from build123d import *

# Parameters (mm, degrees)
SKETCH1_R             = 2.6
BOSS_EXTRUDE1_DEPTH   = 1.6
SKETCH2_R             = 3.45
BOSS_EXTRUDE2_DEPTH   = 1.4
M5X0_8_TAPPED_HOLE1_D = 4.2


with BuildPart() as part:
    # Sketch1 → Boss-Extrude1 (new body)
    with BuildSketch(Plane.XY):
        with BuildLine():
            Line((-2.5, 7.216878365), (2.5, 7.216878365))
            Line((2.5, 7.216878365), (26.315698604, 20.966878365))
            Line((26.315698604, 20.966878365), (29.903623675, 21.701093146))
            ThreePointArc((29.903623675, 21.701093146), (30.819646028, 21.599539147), (31.503382336, 20.981546567))
            Line((31.503382336, 20.981546567), (33.922243506, 16.791956125))
            ThreePointArc((33.922243506, 16.791956125), (34.115572625, 15.890826823), (33.745509792, 15.046751195))
            Line((33.745509792, 15.046751195), (31.315698604, 12.306624327))
            Line((31.315698604, 12.306624327), (7.5, -1.443375673))
            Line((7.5, -1.443375673), (9.220577137, -4.423502692))
            ThreePointArc((9.220577137, -4.423502692), (9.220577137, -5.323502692), (8.441154273, -5.773502692))
            Line((8.441154273, -5.773502692), (-8.441154273, -5.773502692))
            ThreePointArc((-8.441154273, -5.773502692), (-9.220577137, -5.323502692), (-9.220577137, -4.423502692))
            Line((-9.220577137, -4.423502692), (-7.5, -1.443375673))
            Line((-7.5, -1.443375673), (-31.315698604, 12.306624327))
            Line((-31.315698604, 12.306624327), (-33.745509792, 15.046751195))
            ThreePointArc((-33.745509792, 15.046751195), (-34.115572625, 15.890826823), (-33.922243506, 16.791956125))
            Line((-33.922243506, 16.791956125), (-31.503382336, 20.981546567))
            ThreePointArc((-31.503382336, 20.981546567), (-30.819646028, 21.599539147), (-29.903623675, 21.701093146))
            Line((-29.903623675, 21.701093146), (-26.315698604, 20.966878365))
            Line((-26.315698604, 20.966878365), (-2.5, 7.216878365))
        make_face()
        Circle(SKETCH1_R, mode=Mode.SUBTRACT)
    extrude(amount=BOSS_EXTRUDE1_DEPTH)

    # Sketch2 → Boss-Extrude2 (add)
    with BuildSketch(Plane.XY.offset(1.6)):
        with Locations((26.621620912, 15.37)):
            Circle(SKETCH2_R)
        with Locations((9.301112837, 5.37)):
            Circle(SKETCH2_R)
        with Locations((-9.301112837, 5.37)):
            Circle(SKETCH2_R)
        with Locations((-26.621620912, 15.37)):
            Circle(SKETCH2_R)
    extrude(amount=BOSS_EXTRUDE2_DEPTH)

    # M5x0.8 Tapped Hole1 (through all)
    with Locations(Plane.XY.offset(3)):
        with Locations((26.621620912, 15.37), (9.301112837, 5.37), (-9.301112837, 5.37), (-26.621620912, 15.37)):
            Hole(M5X0_8_TAPPED_HOLE1_D / 2)


solid = part.part
Part model, mm, in its own coordinate system. A direction names the side the tool comes from. Give positions to 0.01 mm unless a question says otherwise; leave off trailing zeros. Loops run counter-clockwise (first coordinate to the right, second up) from the corner with the lowest first, then second, coordinate; pieces in that order, holes last.
(1) 3-axis set-ups, long thin cutter, end or side, ignore diameter. For faces 1 (the flat face through (14.241, 13.996, 0.789)), 2 (the cylindrical face through (5.854, 5.522, 2.29)), 3 (the cylindrical face through (-28.561, 14.566, 1.479)): which of +Z, -Z, +X, -X, +Y, -Y reach the whole face in a straight line?
Return value:
face 1: +Z, -Z, +Y
face 2: +Z
face 3: +Z, -Z
(2) Band-saw the part on D-D (y = 5.37). Write the cut outline in (x, z).
Return value:
outline: (-19.3, 0) - (-11.4, 0) - (-11.4, 3) - (-12.75, 3) - (-12.75, 1.6) - (-19.3, 1.6) - close; (-7.2, 0) - (7.2, 0) - (7.2, 3) - (5.85, 3) - (5.85, 1.6) - (-5.85, 1.6) - (-5.85, 3) - (-7.2, 3) - close; (11.4, 0) - (19.3, 0) - (19.3, 1.6) - (12.75, 1.6) - (12.75, 3) - (11.4, 3) - close
(3) Drill centre lines: line 1 along Y through (x, z) = (-8, 0.65); line 2 along X through (y, z) = (14.5, 1.5); line 3 along Y through (x, z) = (0, 1). Where is each one in solid material? Low to high.
Return value:
line 1: y = -5.77 to -2.31, -1.15 to 3.72, 7.02 to 10.39
line 2: x = -33.26 to -28.53, -24.71 to -15.11, 15.11 to 24.71, 28.53 to 33.26
line 3: y = -5.77 to -2.6, 2.6 to 7.22
(4) Pin check, flat tips, straight feed: pin 1 (1 mm diameter, centred on y = 14, z = 2.5, fed in from +X); pin 2 (8.5 mm diameter, centred on x = 0, y = 0, fed in from +Z); pin 3 (0.5 mm diameter, centred on x = -0.5, z = 0.5, fed in from +Y). Stop position of each tip, or through.
Return value:
pin 1: stops at x = 29.96
pin 2: stops at z = 1.6
pin 3: stops at y = 7.22
(5) Pull direction X, two halves, no side cores. Call faces 4 (the cylindrical face through (-12.04, 3.27, 2.29)), 5 (the flat face through (9, 3, 3)), 6 (the flat face through (-32.73, 18.86, 0.79)), 7 (the cylindrical face through (34.117, 15.904, 0.789)): pulls with the +X half, pulls with the -X half, needs draft (parallel to the pull), parting line crosses it, or undercut.
Return value:
face 4: undercut
face 5: needs draft
face 6: pulls with the -X half
face 7: pulls with the +X half
(6) Band-saw the part on B-B (x = 0). Write the cut outline in (y, z), and give its area (3 significant figures).
Return value:
outline: (-5.77, 0) - (-2.6, 0) - (-2.6, 1.6) - (-5.77, 1.6) - close; (2.6, 0) - (7.22, 0) - (7.22, 1.6) - (2.6, 1.6) - close
area: 12.5 mm2
(7) Band-saw the part on A-A (z = 2.45). Write the cut outline in (x, y).
Return value:
outline: circle Ø6.9 at (-26.62, 15.37); circle Ø6.9 at (-9.3, 5.37); circle Ø6.9 at (9.3, 5.37); circle Ø6.9 at (26.62, 15.37); hole circle Ø4.2 at (-26.62, 15.37); hole circle Ø4.2 at (-9.3, 5.37); hole circle Ø4.2 at (9.3, 5.37); hole circle Ø4.2 at (26.62, 15.37)
(8) Band-saw the part on C-C (y = 0). Write the cut outline in (x, z), and give its area (3 significant figures).
Return value:
outline: (-10, 0) - (-2.6, 0) - (-2.6, 1.6) - (-10, 1.6) - close; (2.6, 0) - (10, 0) - (10, 1.6) - (2.6, 1.6) - close
area: 23.7 mm2
